```python
from build123d import *


with BuildPart() as part:
    # Sketch1 → Revolve1 (revolve)
    with BuildSketch(Plane(origin=(0, 0, 0), x_dir=(1, 0, 0), z_dir=(0, 1, 0))):
        with BuildLine():
            Line((8.763, 25.4), (12.7, 101.6))
            ThreePointArc((12.7, 101.6), (9.191372869, 110.791372869), (0, 114.3))
            Line((0, 114.3), (0, 19.05))
            Line((0, 19.05), (6.223, 19.05))
            Line((6.223, 19.05), (6.223, 0))
            Line((6.223, 0), (8.763, 0))
            ThreePointArc((8.763, 0), (10.532289915, 6.35), (8.763, 12.7))
            ThreePointArc((8.763, 12.7), (10.532289915, 19.05), (8.763, 25.4))
        make_face()
    revolve(axis=Axis((0, 0, 810.661063807), (0, 0, -1)))


solid = part.part
```
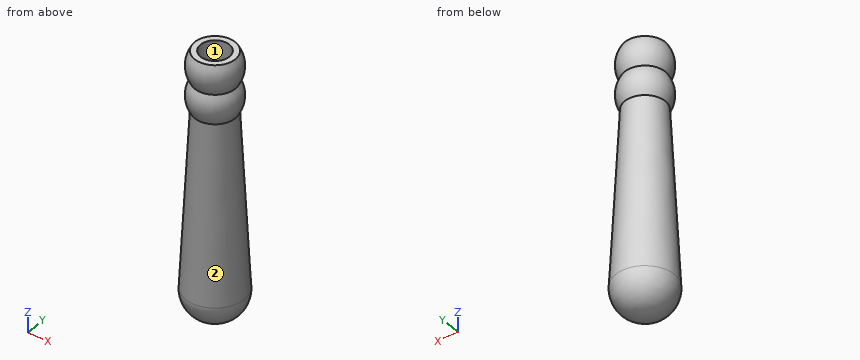
Can you work these out from the model? Positions are in its coordinate system, mm. Face numbers are marked on the shaded views. Coordinates: 2 decimals unless noted, no trailing zeros. Write each loop counter-clockwise with the first axis right and the second up, starting at its lowest first coordinate (ties: lowest second). Pieces come first, ordered by that corner, then holes. Notation, with made-up numbers: (8.25, 45.5) - (48.25, 45.5) arc R22 cw to (48.25, 64.5) - close; hole circle Ø10 at (-14.5, 24). An arc over 180 degrees is marked (long way). Return JSON: item names as keys, results as strings.
Q1. If we section it at A-A (z = -46): Please give me the cut outline in (x, y), then the cut area to 3 significant figures.
Computed values:
{"outline": "circle Ø19.65 at (0, 0)", "area": "303 mm2"}
Q2. Please list where these lines run through material, in increasing order: L1, parallel to Y at x = 0, z = -6.5; L2, parallel to Y at x = 0, z = -4.5; L3, parallel to X at y = 0, z = -8.5. Write a range as from..to.
Computed values:
{"L1": "y = -10.53..-6.22, 6.22..10.53", "L2": "y = -10.39..-6.22, 6.22..10.39", "L3": "x = -10.34..-6.22, 6.22..10.34"}
Q3. I'm going to push flat-ended pins straight in: pin 1 Ø1 at (x, y) = (8.5, -3) entering from -Z; pin 2 Ø3 at (y, z) = (-5, -94) entering from -X; pin 3 Ø10 at (x, y) = (0, -1) entering from +Z. Where does each tip first touch, or does it pass through?
Computed values:
{"pin 1": "stops at z = -111.42", "pin 2": "stops at x = -11.81", "pin 3": "stops at z = -19.05"}
Q4. Thinking about a two-plate mould opening in Z: for the marked faces 1 and 2, which applies, +Z half, -Z half, draft (parallel to the pull), parting line (faces both ways), or undercut?
Computed values:
{"face 1": "draft", "face 2": "undercut"}
